```python
from build123d import *

# Parameters (mm, degrees)
BOSS_EXTRUDE1_DEPTH = 10
FILLET1_R           = 2
SKETCH2_W           = 26.5
SKETCH2_H           = 22
BOSS_EXTRUDE2_DEPTH = 20
CHAMFER1_SIZE       = 15


with BuildPart() as part:
    # Sketch1 → Boss-Extrude1 (new body)
    with BuildSketch(Plane(origin=(0, 0, 0), x_dir=(0, 0, -1), z_dir=(1, 0, 0))):
        Polygon((-26.5, -27.5), (-26.5, -5.5), (-23.5, -5.5), (-23.5, -15.5), (-20.5, -15.5), (-20.5, -12.5), (-17.5, -12.5), (-17.5, -17.5), (-12, -17.5), (-12, -20.5), (-15, -20.5), (-15, -23.5), (0, -23.5), (0, -27.5), align=None)
    extrude(amount=BOSS_EXTRUDE1_DEPTH)

    # Fillet1
    fillet1_edges = [part.edges().sort_by_distance(p)[0] for p in [
        (5, -12.5, 17.5),
        (5, -17.5, 12),
    ]]
    fillet(fillet1_edges, radius=FILLET1_R)

    # Sketch2 → Boss-Extrude2 (add)
    with BuildSketch(Plane.ZY):
        with Locations((13.25, -16.5)):
            Rectangle(SKETCH2_W, SKETCH2_H)
    extrude(amount=BOSS_EXTRUDE2_DEPTH)

    # Chamfer1
    chamfer1_edges = [part.edges().sort_by_distance(p)[0] for p in [
        (-20, -16.5, 26.5),
    ]]
    chamfer(chamfer1_edges, length=CHAMFER1_SIZE)

    # Mirror1: part across plane


with BuildPart() as part_1:
    add(part.part)
    add(part.part.mirror(Plane(origin=(10, -23.5, 0), x_dir=(1, 0, 0), z_dir=(0, 0, 1))))


solid = part_1.part
```
Geometry: final body of the model. Coordinates: model frame, mm. A direction names the side the tool comes from. Round coordinates to 2 decimals unless told otherwise and drop trailing zeros. Loops run counter-clockwise (first coordinate to the right, second up) from the corner with the lowest first, then second, coordinate; pieces in that order, holes last. Notation, with made-up numbers: (21, -5) -> (42, -5) arc R9 cw to (42, 7) -> close; hole circle Ø10 at (-20, 45.25). An arc over 180 degrees is marked (long way). Use one line per item in the form item = value.
Item 1: Draft query along Z for faces 4 (the flat face through (3, -17, 26.5)), 5 (the flat face through (5, -20.5, 13)), 6 (the flat face through (5, -10, -23.5)), 7 (the flat face through (-8, -5.5, 0)). Return one class per face: released by +Z, released by -Z, zero draft, split by the parting line, or undercut.
Evaluation:
face_4 = released by +Z
face_5 = undercut
face_6 = undercut
face_7 = zero draft
Item 2: Contact query for flat-ended pins moving along their axis: pin 1 Ø1 at (x, y) = (-6.5, -21) entering from -Z; pin 2 Ø1 at (x, y) = (-11.5, -11) entering from +Z; pin 3 Ø3.5 at (x, z) = (4.5, -22) entering from +Y; pin 4 Ø1.1 at (x, z) = (6.5, -20) entering from +Y. Output: stop coordinate, or through.
Evaluation:
pin_1 = -25.5
pin_2 = 20.5
pin_3 = -5.5
pin_4 = -12.5
Item 3: Access query for faces 1 (the flat face through (5, -20.5, -13)), 2 (the flat face through (-12.6, -16.7, -18.9)), 3 (the flat face through (5, -16, 17.5)). Directions: +Z, -Z, +X, -X, +Y, -Y. A direction counts if a zero-diameter tool reaches every point of the face in a straight line with its end or side. Return the directions, or none.
Evaluation:
face_1 = +X
face_2 = -Z, -X, +Y, -Y
face_3 = +X, +Y
Item 4: Material intervals for probe 1 along Z at (x, y) = (7.5, -16.75); probe 2 along Z at (x, y) = (5, -7.5); probe 3 along X at (y, z) = (-17.5, 9.5), sorted ascending.
Evaluation:
probe_1 = -26.5 to -17.5, 17.5 to 26.5
probe_2 = -26.5 to -23.5, 23.5 to 26.5
probe_3 = -20 to 0
Item 5: Cut plane B-B on z = 22. Output: boundary loops of the cut face in (x, y).
Evaluation:
outline = (-9.5, -27.5) -> (10, -27.5) -> (10, -15.5) -> (0, -15.5) -> (0, -5.5) -> (-9.5, -5.5) -> close
Item 6: Cut plane D-D on y = -16.25. Output: boundary loops of the cut face in (x, z).
Evaluation:
outline = (-20, -11.5) -> (-5, -26.5) -> (10, -26.5) -> (10, -17.5) -> (0, -17.5) -> (0, 17.5) -> (10, 17.5) -> (10, 26.5) -> (-5, 26.5) -> (-20, 11.5) -> close
Item 7: Cut plane C-C on x = 1.5. Output: boundary loops of the cut face in (y, z), then the cut area to 3 significant figures.
Evaluation:
outline = (-27.5, -26.5) -> (-5.5, -26.5) -> (-5.5, -23.5) -> (-15.5, -23.5) -> (-15.5, -20.5) -> (-12.5, -20.5) -> (-12.5, -19.5) arc R2 ccw to (-14.5, -17.5) -> (-17.5, -17.5) -> (-17.5, -14) arc R2 ccw to (-19.5, -12) -> (-20.5, -12) -> (-20.5, -15) -> (-23.5, -15) -> (-23.5, 15) -> (-20.5, 15) -> (-20.5, 12) -> (-19.5, 12) arc R2 ccw to (-17.5, 14) -> (-17.5, 17.5) -> (-14.5, 17.5) arc R2 ccw to (-12.5, 19.5) -> (-12.5, 20.5) -> (-15.5, 20.5) -> (-15.5, 23.5) -> (-5.5, 23.5) -> (-5.5, 26.5) -> (-27.5, 26.5) -> close
area = 479 mm2
Item 8: Cut plane A-A on y = -7.5. Output: boundary loops of the cut face in (x, z).
Evaluation:
outline = (-20, -11.5) -> (-5, -26.5) -> (10, -26.5) -> (10, -23.5) -> (0, -23.5) -> (0, 23.5) -> (10, 23.5) -> (10, 26.5) -> (-5, 26.5) -> (-20, 11.5) -> close
